```python
from build123d import *

# Parameters (mm, degrees)
F0_W          = 20.0000000001
F0_H          = 40
F0_R          = 2.1
F0_W_2        = 20
F0_H_2        = 5
F1_DEPTH      = 5
F2_START      = 5
F0_W_3        = 50
F2_DEPTH      = 50
F3_START      = 55
F3_DEPTH      = 3
F4_W          = 20
F4_H          = 40
F4_H_2        = 5
F5_DEPTH      = 3
F6_START      = -123
F5_FACE_W     = 20
F5_FACE_H     = 45
F6_DEPTH      = 3
F7_W          = 122
F7_H          = 52
F8_DEPTH      = 5
F8_DEPTH_BACK = 5
F9_DEPTH      = 7.5
F10_W         = 10
F10_H         = 2.5
F11_DEPTH     = 58
F12_W         = 90
F12_H         = 25
F13_DEPTH     = 10


with BuildPart() as f1:
    # F0 (on Front) → F1 (new body)
    with BuildSketch(Plane.XZ):
        with Locations((117.7309190904, 7.2080208344)):
            Rectangle(F0_W, F0_H)
        with Locations((117.7309190904, 6.9580208345)):
            Circle(F0_R, mode=Mode.SUBTRACT)
        with Locations((117.7309190904, 20.4580208344)):
            Circle(F0_R, mode=Mode.SUBTRACT)
        with Locations((117.7309190904, -15.2919791656)):
            Rectangle(F0_W_2, F0_H_2)
    extrude(amount=F1_DEPTH)

    # F0 (on Front) → F2 (join)
    with BuildSketch(Plane.XZ.offset(F2_START)):
        with Locations((82.7309190904, -15.2919791656)):
            Rectangle(F0_W_3, F0_H_2)
        with Locations((152.7309190904, -15.2919791656)):
            Rectangle(F0_W_3, F0_H_2)
        with Locations((117.7309190904, -15.2919791656)):
            Rectangle(F0_W_2, F0_H_2)
    extrude(amount=F2_DEPTH)

    # F0 (on Front) → F3 (join)
    with BuildSketch(Plane.XZ.offset(F3_START)):
        with Locations((117.7309190904, 7.2080208344)):
            Rectangle(F0_W, F0_H)
        with Locations((117.7309190904, 6.9580208345)):
            Circle(F0_R, mode=Mode.SUBTRACT)
        with Locations((117.7309190904, 20.4580208344)):
            Circle(F0_R, mode=Mode.SUBTRACT)
        with Locations((117.7309190904, -15.2919791656)):
            Rectangle(F0_W_2, F0_H_2)
        with Locations((117.7309190904, 20.4580208344)):
            Circle(F0_R)
        with Locations((117.7309190904, 6.9580208345)):
            Circle(F0_R)
    extrude(amount=F3_DEPTH)

    # F4 (on face) → F5 (join)
    with BuildSketch(Plane(origin=(57.7309190904, 0, 0), x_dir=(0, -1, 0), z_dir=(-1, 0, 0))):
        with Locations((30, 7.2080208344)):
            Rectangle(F4_W, F4_H)
        with Locations((30, -15.2919791656)):
            Rectangle(F4_W, F4_H_2)
    extrude(amount=F5_DEPTH)

    # F5_face (on face) → F6 (join)
    with BuildSketch(Plane(origin=(54.7309190904, -30, 4.7080208344), x_dir=(0, -1, 0), z_dir=(-1, 0, 0)).offset(F6_START)):
        Rectangle(F5_FACE_W, F5_FACE_H)
    extrude(amount=-F6_DEPTH)

    # F7 (on face) → F8 (join, two sides)
    with BuildSketch(Plane.XY.offset(-12.7919791656)) as f8_sk:
        with Locations((117.7309190904, -30)):
            Rectangle(F7_W, F7_H)
        Polygon((177.7309190904, -5), (177.7309190904, -20), (177.7309190904, -40), (177.7309190904, -55), (127.7309190904, -55), (107.7309190904, -55), (57.7309190904, -55), (57.7309190904, -40), (57.7309190904, -20), (57.7309190904, -5), (107.7309190904, -5), (127.7309190904, -5), align=None, mode=Mode.SUBTRACT)
    extrude(amount=F8_DEPTH)
    extrude(f8_sk.sketch, amount=-F8_DEPTH_BACK)

    # F9 (add): faces of the model
    f9_faces = [f1.faces().sort_by_distance(p)[0] for p in [
        (117.7309190904, -2.5, 27.2080208344),
        (117.7309190904, -56.5, 27.2080208344),
    ]]
    extrude(f9_faces, amount=F9_DEPTH)

    # F10 (on face) → F11 (cut, through all)
    with BuildSketch(Plane(origin=(0, 0, 0), x_dir=(-1, 0, 0), z_dir=(0, 1, 0))):
        with Locations((-117.7309190904, 31.9580208344)):
            Rectangle(F10_W, F10_H)
    extrude(amount=-F11_DEPTH, mode=Mode.SUBTRACT)

    # F12 (on face) → F13 (cut, through all)
    with BuildSketch(Plane(origin=(0, 0, -17.7919791656), x_dir=(1, 0, 0), z_dir=(0, 0, -1))):
        Polygon((56.7309190904, 4), (68.7309190904, 4), (56.7309190904, 16), align=None)
        Polygon((56.7309190904, 56), (56.7309190904, 44), (68.7309190904, 56), align=None)
        Polygon((166.7309190904, 56), (178.7309190904, 44), (178.7309190904, 56), align=None)
        Polygon((178.7309190904, 16), (166.7309190904, 4), (178.7309190904, 4), align=None)
        with Locations((117.7309190904, 30)):
            Rectangle(F12_W, F12_H)
    extrude(amount=-F13_DEPTH, mode=Mode.SUBTRACT)


solid = f1.part
```
Verification items for the finished model (mm, model axes). A direction names the side the tool comes from. Give positions to 0.01 mm unless a question says otherwise; leave off trailing zeros. Order: outer loops, then holes, each group sorted by start corner. A loop starts at its lowest first (then second) coordinate and runs counter-clockwise, first axis right, second up. Notation, with made-up numbers: (9.5, 85) -> (66.5, 85) arc R29 ccw to (66.5, 107) -> close; hole circle Ø1 at (28.5, -19.5). An arc over 180 degrees is marked (long way). Use a Markdown table: item, result.
1) Section check A-A, the plane x = 138. Record the boundary of the cut face in (y, z).
Results:
| item | result |
|---|---|
| outline | (-56, -17.79) -> (-42.5, -17.79) -> (-42.5, -12.79) -> (-55, -12.79) -> (-55, -7.79) -> (-56, -7.79) -> close; (-17.5, -17.79) -> (-4, -17.79) -> (-4, -7.79) -> (-5, -7.79) -> (-5, -12.79) -> (-17.5, -12.79) -> close |
2) Material ranges on probe 1 along X at (y, z) = (-39, 27); probe 2 along Y at (x, z) = (123.5, 24); probe 3 along X at (y, z) = (-4.5, 31.5), recorded low to high.
Results:
| item | result |
|---|---|
| probe 1 | 54.73 to 57.73, 177.73 to 180.73 |
| probe 2 | -58 to -55, -5 to 0 |
| probe 3 | 107.73 to 112.73, 122.73 to 127.73 |
3) Section check B-B, the plane z = 28.5. Record the boundary of the cut face in (x, y).
Results:
| item | result |
|---|---|
| outline | (107.73, -58) -> (127.73, -58) -> (127.73, -55) -> (107.73, -55) -> close; (107.73, -5) -> (127.73, -5) -> (127.73, 0) -> (107.73, 0) -> close |
4) Section check C-C, the plane y = -29. Record the boundary of the cut face in (x, z).
Results:
| item | result |
|---|---|
| outline | (54.73, -17.79) -> (72.73, -17.79) -> (72.73, -12.79) -> (57.73, -12.79) -> (57.73, 27.21) -> (54.73, 27.21) -> close; (162.73, -17.79) -> (180.73, -17.79) -> (180.73, 27.21) -> (177.73, 27.21) -> (177.73, -12.79) -> (162.73, -12.79) -> close |
5) Tool access check on faces 1 (the flat face through (117, -42.5, -15)), 2 (the flat face through (56.731, -18, -13)), 3 (the flat face through (147, -56, -13)), 4 (the flat face through (119, -46, -12.792)). Record the directions out of +Z, -Z, +X, -X, +Y, -Y that give a thin tool (end or side, any length) a straight path to the whole face; none if there is none.
Results:
| item | result |
|---|---|
| face 1 | +Z, -Z |
| face 2 | +Z, -Z, -X, +Y |
| face 3 | +Z, -Z, +X, -Y |
| face 4 | +Z |
6) Section check D-D, the plane z = -6. Record the boundary of the cut face in (x, y).
Results:
| item | result |
|---|---|
| outline | (54.73, -40) -> (57.73, -40) -> (57.73, -20) -> (54.73, -20) -> close; (107.73, -58) -> (127.73, -58) -> (127.73, -55) -> (107.73, -55) -> close; (107.73, -5) -> (127.73, -5) -> (127.73, 0) -> (107.73, 0) -> close; (177.73, -40) -> (180.73, -40) -> (180.73, -20) -> (177.73, -20) -> close |
7) Depth check by flat-ended pin: pin 1 Ø3 at (x, z) = (85.5, -11) entering from +Y; pin 2 Ø3 at (x, y) = (125.5, -9) entering from +Z; pin 3 Ø5.5 at (y, z) = (-2, 10.5) entering from +X. Enter the tip coordinate at first touch or a pass-through.
Results:
| item | result |
|---|---|
| pin 1 | y = -4 |
| pin 2 | z = -12.79 |
| pin 3 | x = 127.73 |
8) Mould release check, pull along Y, two halves, no side actions. Record for faces 5 (the flat face through (118, -2, 34.708)), 6 (the flat face through (118, -55, 6)), 7 (the flat face through (172.65, -50.08, -13.97)): pulls with the +Y half, pulls with the -Y half, needs draft (parallel to the pull), parting line crosses it, or undercut.
Results:
| item | result |
|---|---|
| face 5 | needs draft |
| face 6 | undercut |
| face 7 | pulls with the -Y half |
